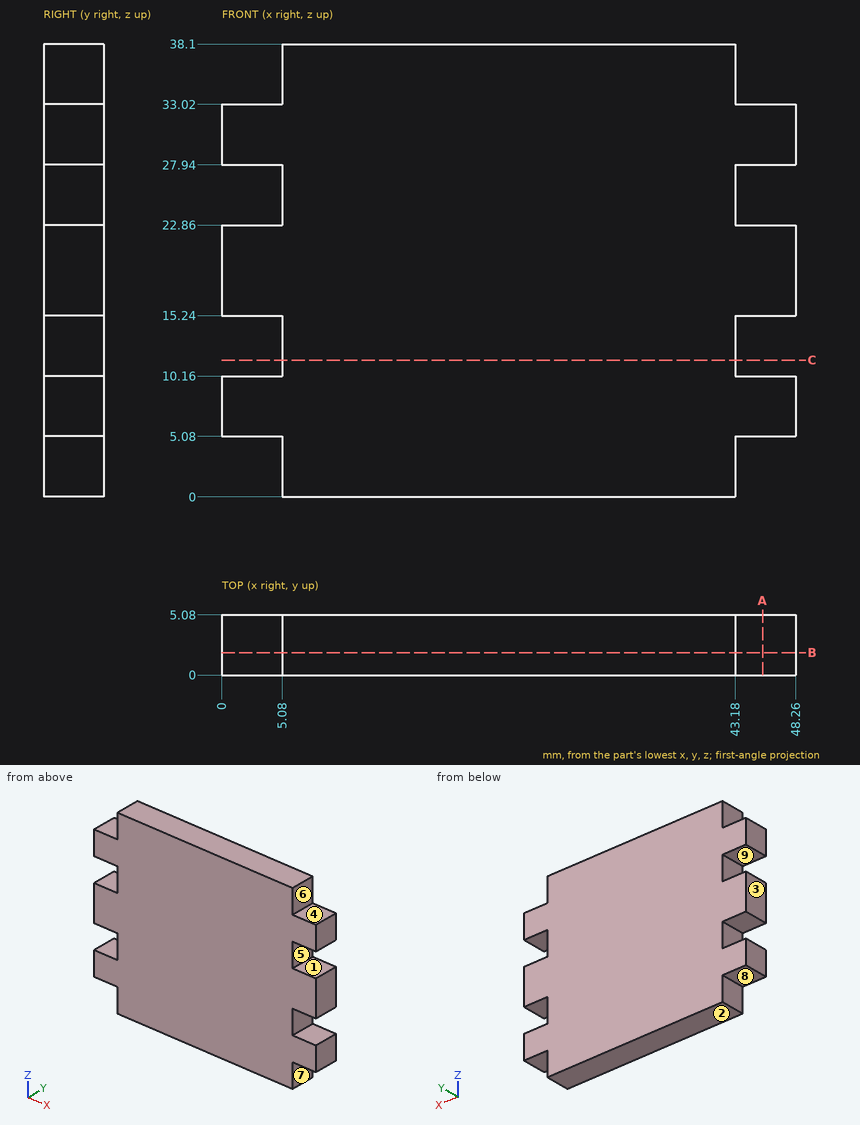
Job drawing, mm, ordinate dimensions from the low corner. One solid piece. A direction names the side the tool comes from. Round coordinates to 2 decimals unless told otherwise and drop trailing zeros. Loops run counter-clockwise (first coordinate to the right, second up) from the corner with the lowest first, then second, coordinate; pieces in that order, holes last.
Item 1: Cut at C-C, the plane z = 11.5. Give the cut face in (x, y).
Item 2: Cut at B-B, the plane y = 1.9. Give the cut face in (x, z).
Item 3: Drop flat-ended pins along their axis: P1, Ø2, axis at x = 40, z = 13.5, coming from the -Y side; P2, Ø2.5, axis at x = 46, y = 3, coming from the -Z side; P3, Ø1.5, axis at x = 2, y = 3.5, coming from the +Z side; P4, Ø1.5, axis at y = 3, z = 3, coming from the +X side. Give the stop position or say it passes through.
Item 4: Drill centre lines: line 1 (Z direction, x = 2, y = 3.75); line 2 (X direction, y = 3.1, z = 26). Where is each one in solid material? Low to high.
Item 5: Mould opens along Z. For the marked faces 1, 2, 3 and 4 say: +Z half, -Z half, draft (parallel to the pull), parting line (faces both ways), or undercut.
Item 6: 3-axis set-ups, long thin cutter, end or side, ignore diameter. For the marked faces 5, 6, 7, 8 and 9: which of +Z, -Z, +X, -X, +Y, -Y reach the whole face in a straight line?
Item 7: Cut at A-A, the plane x = 45.5. Give the cut face in (y, z).
A:
1. outline: (5.08, 0) - (43.18, 0) - (43.18, 5.08) - (5.08, 5.08) - close
2. outline: (0, 5.08) - (5.08, 5.08) - (5.08, 0) - (43.18, 0) - (43.18, 5.08) - (48.26, 5.08) - (48.26, 10.16) - (43.18, 10.16) - (43.18, 15.24) - (48.26, 15.24) - (48.26, 22.86) - (43.18, 22.86) - (43.18, 27.94) - (48.26, 27.94) - (48.26, 33.02) - (43.18, 33.02) - (43.18, 38.1) - (5.08, 38.1) - (5.08, 33.02) - (0, 33.02) - (0, 27.94) - (5.08, 27.94) - (5.08, 22.86) - (0, 22.86) - (0, 15.24) - (5.08, 15.24) - (5.08, 10.16) - (0, 10.16) - close
3. P1: stops at y = 0
3. P2: stops at z = 5.08
3. P3: stops at z = 33.02
3. P4: stops at x = 43.18
4. line 1: z = 5.08 to 10.16, 15.24 to 22.86, 27.94 to 33.02
4. line 2: x = 5.08 to 43.18
5. face 1: undercut
5. face 2: -Z half
5. face 3: draft
5. face 4: +Z half
6. face 5: +X, +Y, -Y
6. face 6: +Z, +X, +Y, -Y
6. face 7: -Z, +X, +Y, -Y
6. face 8: -Z, -X, +Y, -Y
6. face 9: -X, +Y, -Y
7. outline: (0, 5.08) - (5.08, 5.08) - (5.08, 10.16) - (0, 10.16) - close; (0, 15.24) - (5.08, 15.24) - (5.08, 22.86) - (0, 22.86) - close; (0, 27.94) - (5.08, 27.94) - (5.08, 33.02) - (0, 33.02) - close
